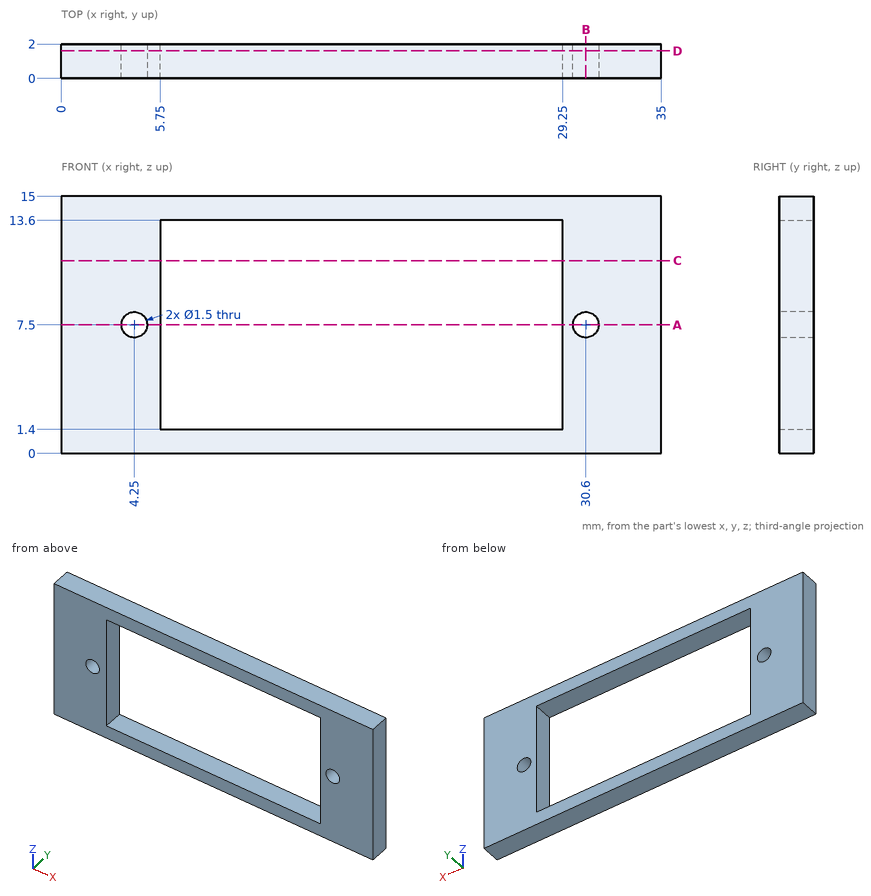
Input: dimensioned drawing with shaded views. Units: mm. Origin: part minimum x, y, z. Give positions to 0.01 mm unless a question says otherwise; leave off trailing zeros. Write each loop counter-clockwise with the first axis right and the second up, starting at its lowest first coordinate (ties: lowest second). Pieces come first, ordered by that corner, then holes. Notation, with made-up numbers: (86, -20) -> (124, -20) arc R13 cw to (124, -4) -> close; hole circle Ø1 at (-2.75, 48.25). An arc over 180 degrees is marked (long way). Answer as a JSON object with one key per item and string values.
1. Cut plane D-D on y = 1.6. Output: boundary loops of the cut face in (x, z), and give its area (3 significant figures).
Ans:
{"outline": "(0, 0) -> (35, 0) -> (35, 15) -> (0, 15) -> close; hole circle Ø1.5 at (4.25, 7.5); hole (5.75, 1.4) -> (29.25, 1.4) -> (29.25, 13.6) -> (5.75, 13.6) -> close; hole circle Ø1.5 at (30.6, 7.5)", "area": "235 mm^2"}
2. Cut plane B-B on x = 30.6. Output: boundary loops of the cut face in (y, z).
Ans:
{"outline": "(0, 0) -> (2, 0) -> (2, 6.75) -> (0, 6.75) -> close; (0, 8.25) -> (2, 8.25) -> (2, 15) -> (0, 15) -> close"}
3. Ray query, probe 1 along Z at (x, y) = (24, 0.4); probe 2 along X at (y, z) = (0.85, 4); probe 3 along Z at (x, y) = (30.6, 0.6). Return the intervals inside material, ascending. Write a range as from..to.
Ans:
{"probe 1": "z = 0..1.4, 13.6..15", "probe 2": "x = 0..5.75, 29.25..35", "probe 3": "z = 0..6.75, 8.25..15"}
4. Cut plane A-A on z = 7.5. Output: boundary loops of the cut face in (x, y).
Ans:
{"outline": "(0, 0) -> (3.5, 0) -> (3.5, 2) -> (0, 2) -> close; (5, 0) -> (5.75, 0) -> (5.75, 2) -> (5, 2) -> close; (29.25, 0) -> (29.85, 0) -> (29.85, 2) -> (29.25, 2) -> close; (31.35, 0) -> (35, 0) -> (35, 2) -> (31.35, 2) -> close"}
5. Cut plane C-C on z = 11.25. Output: boundary loops of the cut face in (x, y).
Ans:
{"outline": "(0, 0) -> (5.75, 0) -> (5.75, 2) -> (0, 2) -> close; (29.25, 0) -> (35, 0) -> (35, 2) -> (29.25, 2) -> close"}
